from build123d import *

# Parameters (mm, degrees)
SKETCH2_W             = 202
SKETCH2_H             = 13.5
BASE_FLANGE1_DEPTH    = 1
EDGE_FLANGE1_DEPTH    = 202
SWEPT_FLANGE2_DEPTH   = 202
SWEPT_FLANGE2_2_DEPTH = 202
EDGE_FLANGE2_DEPTH    = 202
EDGE_FLANGE3_DEPTH    = 48.9


# Read off the part's stored shape, not the designer's step: Swept Flange2
# Sheet-metal steps are written as plain solids
with BuildPart() as part:
    # Sketch2 → Base-Flange1 (new body)
    with BuildSketch(Plane(origin=(0, 0, 0), x_dir=(1, 0, 0), z_dir=(0, 1, 0))):
        with Locations((101, 6.75)):
            Rectangle(SKETCH2_W, SKETCH2_H)
    extrude(amount=-BASE_FLANGE1_DEPTH)

    # Edge-Flange1 section (across the edge) → Edge-Flange1 (add)
    with BuildSketch(Plane(origin=(202, 0, -13.6), x_dir=(0, 0, 1), z_dir=(-1, 0, 0))):
        with BuildLine():
            Line((-1, 0.1), (-1, 49))
            Line((-1, 49), (0, 49))
            Line((0, 49), (0, 0.1))
            ThreePointArc((0, 0.1), (0.029289322, 0.029289322), (0.1, 0))
            Line((0.1, 0), (0.1, -1))
            ThreePointArc((0.1, -1), (-0.677817459, -0.677817459), (-1, 0.1))
        make_face()
    extrude(amount=EDGE_FLANGE1_DEPTH)

    # Swept Flange2 outline → Swept Flange2 (cut)
    with BuildSketch(Plane.YZ):
        with BuildLine():
            ThreePointArc((-1, -0.266145802), (-0.991798775, -0.132073302), (-0.967317391, 0))
            Line((-0.967317391, 0), (-1, 0))
            Line((-1, 0), (-1, -0.266145802))
        make_face()
    extrude(amount=SWEPT_FLANGE2_DEPTH, mode=Mode.SUBTRACT)

    # Swept Flange2 2 outline → Swept Flange2 2 (add)
    with BuildSketch(Plane.YZ):
        with BuildLine():
            Line((0, 21.5), (-1, 21.5))
            Line((-1, 21.5), (-1, 8.266145802))
            ThreePointArc((-1, 8.266145802), (-0.970971133, 8.015106296), (-0.885416667, 7.777316595))
            ThreePointArc((-0.885416667, 7.777316595), (0, 4), (-0.885416667, 0.222683405))
            ThreePointArc((-0.885416667, 0.222683405), (-0.932388615, 0.113556382), (-0.967317391, 0))
            Line((-0.967317391, 0), (0, 0))
            Line((0, 0), (0, -0.266145802))
            ThreePointArc((0, -0.266145802), (0.002638988, -0.243324029), (0.010416667, -0.221706783))
            ThreePointArc((0.010416667, -0.221706783), (1, 4), (0.010416667, 8.221706783))
            ThreePointArc((0.010416667, 8.221706783), (0.002638988, 8.243324029), (0, 8.266145802))
            Line((0, 8.266145802), (0, 21.5))
        make_face()
    extrude(amount=SWEPT_FLANGE2_2_DEPTH)

    # Edge-Flange2 section (across the edge) → Edge-Flange2 (add)
    with BuildSketch(Plane(origin=(0, 0, 21.6), x_dir=(0, 0, -1), z_dir=(1, 0, 0))):
        with BuildLine():
            Line((-1, 0.1), (-1, 49))
            Line((-1, 49), (0, 49))
            Line((0, 49), (0, 0.1))
            ThreePointArc((0, 0.1), (0.029289322, 0.029289322), (0.1, 0))
            Line((0.1, 0), (0.1, -1))
            ThreePointArc((0.1, -1), (-0.677817459, -0.677817459), (-1, 0.1))
        make_face()
    extrude(amount=EDGE_FLANGE2_DEPTH)

    # Edge-Flange3 section (across the edge) → Edge-Flange3 (add)
    with BuildSketch(Plane(origin=(202.1, 49, 21.6), x_dir=(-1, 0, 0), z_dir=(0, -1, 0))):
        with BuildLine():
            Line((-1, 0.1), (-1, 36.2))
            Line((-1, 36.2), (0, 36.2))
            Line((0, 36.2), (0, 0.1))
            ThreePointArc((0, 0.1), (0.029289322, 0.029289322), (0.1, 0))
            Line((0.1, 0), (0.1, -1))
            ThreePointArc((0.1, -1), (-0.677817459, -0.677817459), (-1, 0.1))
        make_face()
    extrude(amount=EDGE_FLANGE3_DEPTH)


solid = part.part
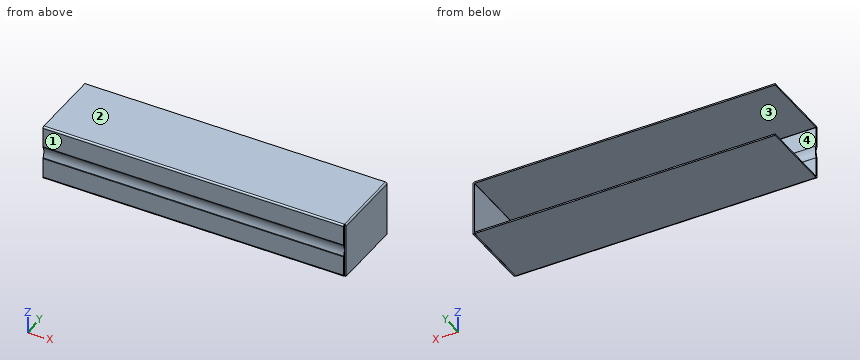
The listing builds one solid part. Answer for the finished solid, in the listing's coordinates (mm). Face numbers are marked on the shaded views. Coordinates: 2 decimals unless noted, no trailing zeros. Loops run counter-clockwise (first coordinate to the right, second up) from the corner with the lowest first, then second, coordinate; pieces in that order, holes last.
1) Find section A-A on y = 28.5. Write down the section's boundary in (x, z), then the cut area to 3 significant figures.
2) Find the intervals of material crossed by L1, parallel to Z at x = 116, y = 18; L2, parallel to X at y = 16, z = -4.5; L3, parallel to Y at x = 176, z = 0, in increasing order.
3) Determine the mould class of the marked faces 1, 2, 3 and 4 for opening direction Z: pulls with the +Z half, pulls with the -Z half, needs draft (parallel to the pull), parting line crosses it, or undercut.
4) Find section C-C on x = 135.5. Write down the section's boundary in (y, z).
5) Find section B-B on z = 12.5. Write down the section's boundary in (x, y), then the cut area to 3 significant figures.
6) Flat-ended cylindrical pins translate along their axes: pin 1 Ø12 at (x, z) = (148, -3) entering from +Y; pin 2 Ø6 at (y, z) = (29.5, 15.5) entering from -X; pin 3 Ø12 at (x, z) = (135, -5.5) entering from +Y. Find the tip coordinate at first contact, or state that the pin passes through.
Values:
1. outline: (0, -14.6) - (202, -14.6) - (202, -13.6) - (0, -13.6) - close; (0, 21.6) - (202, 21.6) arc R0.1 cw to (202.1, 21.5) - (202.1, -14.6) - (203.1, -14.6) - (203.1, 21.5) arc R1.1 ccw to (202, 22.6) - (0, 22.6) - close
1. area: 441 mm2
2. L1: z = -14.6 to -13.6, 21.6 to 22.6
2. L2: x = 202.1 to 203.1
2. L3: y = -0.97 to 0.12
3. face 1: needs draft
3. face 2: pulls with the +Z half
3. face 3: undercut
3. face 4: undercut
4. outline: (-1, -13.5) arc R1.1 ccw to (0.1, -14.6) - (49, -14.6) - (49, -13.6) - (0.1, -13.6) arc R0.1 cw to (0, -13.5) - (0, -0.27) arc R0.1 cw to (0.01, -0.22) arc R9.5 ccw to (0.01, 8.22) arc R0.1 cw to (0, 8.27) - (0, 21.5) arc R0.1 cw to (0.1, 21.6) - (49, 21.6) - (49, 22.6) - (0.1, 22.6) arc R1.1 ccw to (-1, 21.5) - (-1, 8.27) arc R1.1 ccw to (-0.89, 7.78) arc R8.5 cw to (-0.89, 0.22) arc R1.1 ccw to (-1, -0.27) - close
5. outline: (0, -1) - (202, -1) - (202, 0) - (0, 0) - close; (202.1, 0.1) - (203.1, 0.1) - (203.1, 49) - (202.1, 49) - close
5. area: 251 mm2
6. pin 1: stops at y = 0.95
6. pin 2: stops at x = 202.1
6. pin 3: stops at y = 0.33
